Source: CAD feature listing. Evaluate the final solid. Frame: model axes, mm. Face numbers are marked on the shaded views. A direction names the side the tool comes from. Coordinates: 2 decimals unless noted, no trailing zeros. Order: outer loops, then holes, each group sorted by start corner. A loop starts at its lowest first (then second) coordinate and runs counter-clockwise, first axis right, second up. Notation, with made-up numbers: (48, 24.5) - (73, 24.5) arc R13 cw to (73, 32.5) - close; hole circle Ø2 at (-27, 89.25). An arc over 180 degrees is marked (long way). One line per question, with ' | ' between items.
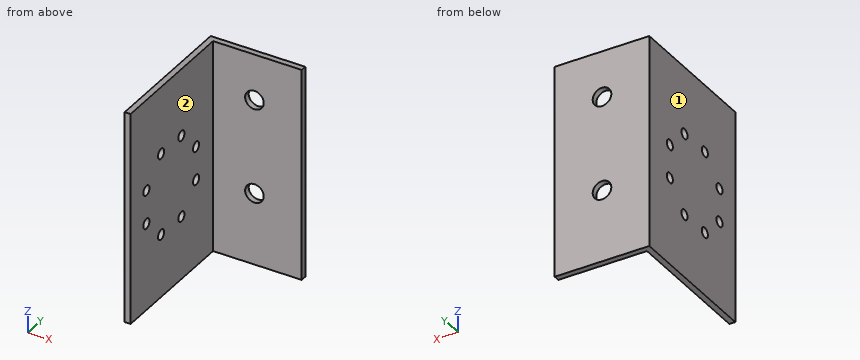
from build123d import *

# Parameters (mm, degrees)
BOSS_EXTRUDE1_DEPTH = 57.15
SKETCH3_R           = 1.35
CUT_EXTRUDE1_DEPTH  = 2.5875
SKETCH2_R           = 2.5
CUT_EXTRUDE2_DEPTH  = 2.5875


with BuildPart() as part:
    # Sketch1 → Boss-Extrude1 (new body)
    with BuildSketch(Plane.XY):
        Polygon((-0.251653512, 27.381273354), (-25.651653512, 27.381273354), (-25.651653512, -10.718726646), (-24.064153512, -10.718726646), (-24.064153512, 25.793773354), (-0.251653512, 25.793773354), align=None)
    extrude(amount=BOSS_EXTRUDE1_DEPTH)

    # Sketch3 → Cut-Extrude1 (cut, through all)
    with BuildSketch(Plane(origin=(-24.064153512, 0, 0), x_dir=(0, 0, -1), z_dir=(1, 0, 0))):
        with Locations((-32.5, 18.281273354)):
            Circle(SKETCH3_R)
        with Locations((-23.5, 18.281273354)):
            Circle(SKETCH3_R)
        with Locations((-17, 11.781273354)):
            Circle(SKETCH3_R)
        with Locations((-17, 2.781273354)):
            Circle(SKETCH3_R)
        with Locations((-23.5, -3.718726646)):
            Circle(SKETCH3_R)
        with Locations((-32.5, -3.718726646)):
            Circle(SKETCH3_R)
        with Locations((-39, 2.781273354)):
            Circle(SKETCH3_R)
        with Locations((-39, 11.781273354)):
            Circle(SKETCH3_R)
    extrude(amount=-CUT_EXTRUDE1_DEPTH, mode=Mode.SUBTRACT)

    # Sketch2 → Cut-Extrude2 (cut, through all)
    with BuildSketch(Plane.XZ.offset(-25.793773354)):
        with Locations((-12.951653512, 44.762965599)):
            Circle(SKETCH2_R)
        with Locations((-12.951653512, 19.362965599)):
            Circle(SKETCH2_R)
    extrude(amount=-CUT_EXTRUDE2_DEPTH, mode=Mode.SUBTRACT)


solid = part.part
(1) Cut plane B-B (x = -12). Return the cut outline in (y, z).
Taken from the geometry:
outline: (25.79, 0) - (27.38, 0) - (27.38, 17.05) - (25.79, 17.05) - close; (25.79, 21.67) - (27.38, 21.67) - (27.38, 42.45) - (25.79, 42.45) - close; (25.79, 47.07) - (27.38, 47.07) - (27.38, 57.15) - (25.79, 57.15) - close
(2) Pin query (flat end, axial travel): P1, Ø8, axis at y = 21, z = 16.5, coming from the +X side; P2, Ø3.5, axis at y = 18.28, z = 23.5, coming from the -X side; P3, Ø6, axis at x = -12.95, z = 19.36, coming from the -Y side. Return the tip coordinate at first contact, or that it passes through.
Taken from the geometry:
P1: stops at x = -24.06 | P2: stops at x = -25.65 | P3: stops at y = 25.79
(3) Material intervals for L1, parallel to Y at x = -24.6, z = 32.5; L2, parallel to Y at x = -25.15, z = 39; L3, parallel to Y at x = -9, z = 17.5, sorted ascending. Write a range as from..to.
Taken from the geometry:
L1: y = -10.72..-5.07, -2.37..16.93, 19.63..27.38 | L2: y = -10.72..1.43, 4.13..10.43, 13.13..27.38 | L3: y = 25.79..27.38
(4) Cut plane C-C (z = 6). Return the cut outline in (x, y).
Taken from the geometry:
outline: (-25.65, -10.72) - (-24.06, -10.72) - (-24.06, 25.79) - (-0.25, 25.79) - (-0.25, 27.38) - (-25.65, 27.38) - close
(5) Set-up query: the marked faces 1 and 2. Return all of +Z, -Z, +X, -X, +Y, -Y with unobstructed straight access to the full face (end or side cutting, diameter ignored); none if empty.
Taken from the geometry:
face 1: +Z, -Z, -X, +Y, -Y | face 2: +Z, -Z, +X, -Y
(6) Cut plane D-D (z = 46). Return the cut outline in (x, y).
Taken from the geometry:
outline: (-25.65, -10.72) - (-24.06, -10.72) - (-24.06, 25.79) - (-15.12, 25.79) - (-15.12, 27.38) - (-25.65, 27.38) - close; (-10.78, 25.79) - (-0.25, 25.79) - (-0.25, 27.38) - (-10.78, 27.38) - close
(7) Cut plane A-A (z = 32.5). Return the cut outline in (x, y), and give its area (3 significant figures).
Taken from the geometry:
outline: (-25.65, -10.72) - (-24.06, -10.72) - (-24.06, -5.07) - (-25.65, -5.07) - close; (-25.65, -2.37) - (-24.06, -2.37) - (-24.06, 16.93) - (-25.65, 16.93) - close; (-25.65, 19.63) - (-24.06, 19.63) - (-24.06, 25.79) - (-0.25, 25.79) - (-0.25, 27.38) - (-25.65, 27.38) - close | area: 89.7 mm²
